Autodesk Inventor part; units mm, degrees
ref_plane "YZ Plane" through (0, 0, 0) normal (1, 0, 0) x (0, 1, 0)
ref_plane "XZ Plane" through (0, 0, 0) normal (0, 1, 0) x (-1, 0, 0)
ref_plane "XY Plane" through (0, 0, 0) normal (0, 0, 1) x (1, 0, 0)
sketch "Sketch1" plane through (0, 0, 0) normal (0, 0, 1) x (1, 0, 0)
  line L0 (-12.7, -6.35) -> (12.7, -6.35) construction
  line L1 (12.7, -6.35) -> (12.7, 6.35) construction
  line L2 (12.7, 6.35) -> (-12.7, 6.35) construction
  line L3 (-12.7, 6.35) -> (-12.7, -6.35) construction
  line L4 (-12.7, -6.35) -> (12.7, 6.35) construction
  line L5 (12.7, -6.35) -> (-12.7, 6.35) construction
  circle A0 centre (0, 0) radius 11
  circle A1 centre (-12.7, 6.35) radius 1.5875
  circle A2 centre (12.7, 6.35) radius 1.5875
  circle A3 centre (-12.7, -6.35) radius 1.5875
  circle A4 centre (12.7, -6.35) radius 1.5875
  line L6 (-15.875, -9.525) -> (15.875, -9.525)
  line L7 (15.875, -9.525) -> (15.875, 9.525)
  line L8 (15.875, 9.525) -> (-15.875, 9.525)
  line L9 (-15.875, 9.525) -> (-15.875, -9.525)
  line L10 (-15.875, -9.525) -> (15.875, 9.525) construction
  line L11 (15.875, -9.525) -> (-15.875, 9.525) construction
  line L12 (9.525, -12.7) -> (-9.525, -12.7)
  line L13 (-9.525, -12.7) -> (-9.525, 12.7)
  line L14 (-9.525, 12.7) -> (9.525, 12.7)
  line L15 (9.525, 12.7) -> (9.525, -12.7)
  line L16 (9.525, -12.7) -> (-9.525, 12.7) construction
  line L17 (-9.525, -12.7) -> (9.525, 12.7) construction
  point P0 (-9.525, 9.525)
  point P1 (-5.5022, 9.525)
  point P2 (5.5022, 9.525)
  point P3 (9.525, 9.525)
  point P4 (9.525, -9.525)
  point P5 (5.5022, -9.525)
  point P6 (-5.5022, -9.525)
  point P7 (-9.525, -9.525)
  dimension "d0" = 25.4
  dimension "d1" = 12.7
  dimension "d2" = 22
  dimension "d3" = 3.175
  dimension "d6" = 25.4
  dimension "d9" = 12.7
  dimension "d12" = 31.75
  dimension "d13" = 19.05
  dimension "d42" = 19.05
  dimension "d43" = 25.4
extrude "Extrusion1" add sketch "Sketch1" along normal blind 13.625 contours A0 L15 L8 L7 L6 | A0 L8 L15 | L15 L6 A0 | A0 L8 L13 L14 L15 | L6 L15 L12 L13 A0 | A0 L13 L8 | L6 L13 A0 | A0 L13 L6 L9 L8
ref_plane "Work Plane1" through (-15.875, -6.35, 0) normal (0, -1, 0) x (1, 0, 0)
sketch "Sketch2" plane through (-15.875, -9.525, 0) normal (0, -1, 0) x (1, 0, 0)
  line L0 (0, 0) -> (0, 13.625)
  line L1 (0, 0) -> (-9.525, 0)
  line L2 (-9.525, 0) -> (-9.525, 9.525)
  line L3 (-9.525, 9.525) -> (0, 9.525)
  line L4 (0, 9.525) -> (0, 0)
  line L5 (-9.525, 9.525) -> (0, 0) construction
  circle A0 centre (-4.7625, 4.7625) radius 3.302
  line L6 (15.875, 0) -> (15.875, -6.35) construction
  line L7 (31.75, 0) -> (41.275, 0)
  line L8 (41.275, 0) -> (41.275, 9.525)
  line L9 (41.275, 9.525) -> (31.75, 9.525)
  line L10 (31.75, 9.525) -> (31.75, 0)
  line L11 (41.275, 9.525) -> (31.75, 0) construction
  circle A1 centre (36.5125, 4.7625) radius 3.302
  point P0 (0, 9.525)
  dimension "d38" = 9.525
  dimension "d39" = 9.525
  dimension "d40" = 6.604
  dimension "d41" = 6.35
extrude "Extrusion2" add sketch "Sketch2" against normal blind 19.05
chamfer "Chamfer2" distance 4.1 distance2 9.525 1 edges at (-15.875, 0, 9.525) measured on face at (-15.875, 3.175, 12.2583)
chamfer "Chamfer3" distance 4.1 distance2 9.525 1 edges at (15.875, 0, 9.525) measured on face at (15.875, -3.175, 12.2583)
fillet "Fillet3" radius 1.5875 4 edges at (9.525, -12.7, 6.8125) (-9.525, -12.7, 6.8125) (-9.525, 12.7, 6.8125) (9.525, 12.7, 6.8125)
equation "\"d6\" = d0"
equation "\"d9\" = d1"
properties part number "Motor Sleeve" material "UHMW, White"
Input: part model. Units: mm. Frame: model coordinates. A direction names the side the tool comes from. Give positions to 0.01 mm unless a question says otherwise; leave off trailing zeros. Order: outer loops, then holes, each group sorted by start corner. A loop starts at its lowest first (then second) coordinate and runs counter-clockwise, first axis right, second up. Notation, with made-up numbers: M 35.25,51 L 83.25,51 A26 ccw 83.25,73 Z; hole C 83,41.5 d5. An arc over 180 degrees is marked long. Return JSON: item names as keys, results as strings.
1) Section query A-A on y = 0. Count the separate pieces of the cut face and the enclosed holes in it, and give its area (3 significant figures).
Taken from the geometry:
{"separate pieces": "2", "enclosed holes": "2", "area": "285 mm2"}
2) Contact query for flat-ended pins moving along their axis: pin 1 (5 mm diameter, centred on y = 1, z = 11.5, fed in from -X); pin 2 (7.5 mm diameter, centred on x = -20.64, z = 4.76, fed in from +Y) (3 decimals); pin 3 (4 mm diameter, centred on x = -17.5, z = 5.5, fed in from -Y) (3 decimals); pin 4 (0.5 mm diameter, centred on y = 10, z = 8.5, fed in from -X) (3 decimals). Output: stop coordinate, or through.
Taken from the geometry:
{"pin 1": "stops at x = -25.4", "pin 2": "stops at y = 9.525", "pin 3": "stops at y = -9.525", "pin 4": "stops at x = -9.525"}
3) Access query for faces 5 (the face through (-9.525, -10, 7)), 6 (the face through (-9.525, 10, 7)), 7 (the face through (9.525, -10, 7)). Directions: +Z, -Z, +X, -X, +Y, -Y. A direction counts if a zero-diameter tool reaches every point of the face in a straight line with its end or side. Return the directions, or none.
Taken from the geometry:
{"face 5": "+Z, -Z, -X, -Y", "face 6": "+Z, -Z, -X, +Y", "face 7": "+Z, -Z, +X, -Y"}
4) Mould query, pull axis Y, two halves, no side actions, for faces 1 (the face through (-2.38, 10.74, 6.72)), 2 (the face through (-11, 3, 13.625)), 3 (the face through (16, -9.525, 7)), 4 (the face through (-11.234, -5.742, 6.717)). Classes: released by +Y, released by -Y, zero draft, split by the parting line, or undercut.
Taken from the geometry:
{"face 1": "undercut", "face 2": "zero draft", "face 3": "released by -Y", "face 4": "undercut"}
5) Section query B-B on x = 12.7. Output: boundary loops of the cut face in (y, z) (1 decimal).
Taken from the geometry:
{"outline": "M -9.5,0 L -7.9,0 L -7.9,13.6 L -9.5,13.6 Z; M -4.8,0 L 4.8,0 L 4.8,13.6 L -4.8,13.6 Z; M 7.9,0 L 9.5,0 L 9.5,13.6 L 7.9,13.6 Z"}
6) Line query: L1, parallel to Y at x = 12.7, z = 5 (1 decimal); L2, parallel to X at y = -1.5, z = 4.25; L3, parallel to X at y = 7.5, z = 3. Output: solid intervals per line, ascending. Write a range as [from, to].
Taken from the geometry:
{"L1": "y = [-9.5, -7.9], [-4.8, 4.8], [7.9, 9.5]", "L2": "x = [-25.4, -23.9], [-17.38, -10.9], [10.9, 17.38], [23.9, 25.4]", "L3": "x = [-25.4, -23.43], [-17.85, -13.79], [-11.61, -8.05], [8.05, 11.61], [13.79, 17.85], [23.43, 25.4]"}
